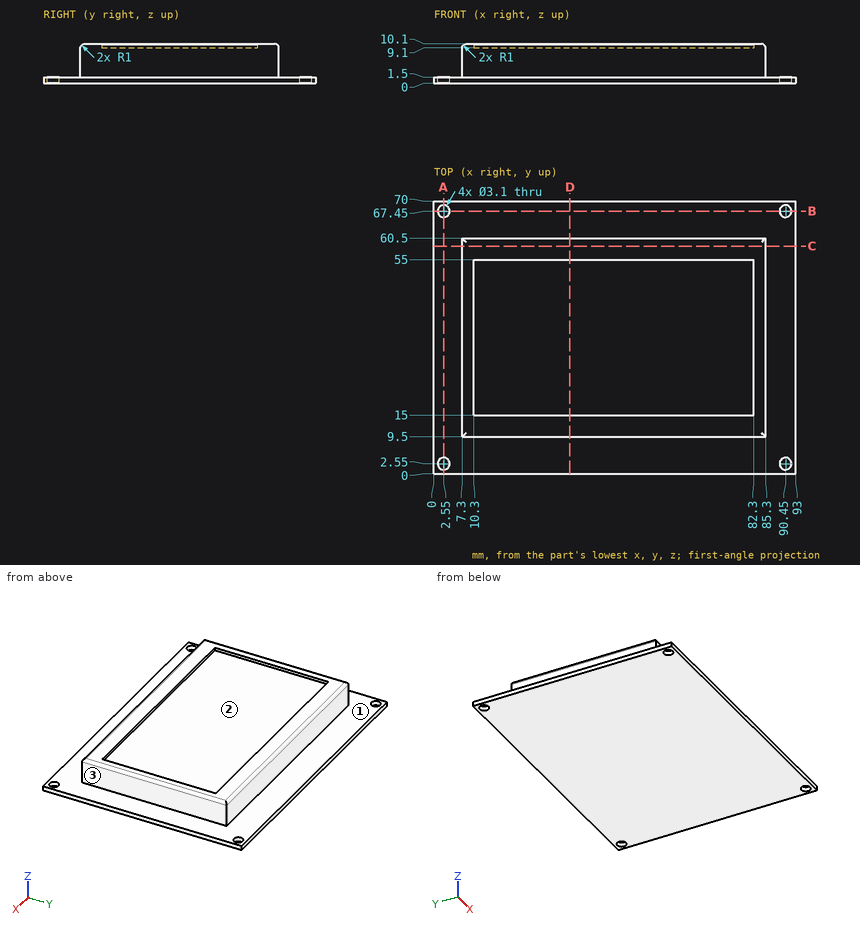
Job drawing, mm, ordinate dimensions from the low corner. One solid piece. Give positions to 0.01 mm unless a question says otherwise; leave off trailing zeros. Order: outer loops, then holes, each group sorted by start corner. A loop starts at its lowest first (then second) coordinate and runs counter-clockwise, first axis right, second up. Notation, with made-up numbers: (-1.75, -12.75) - (31.25, -12.75) arc R29 cw to (31.25, 25.25) - close; hole circle Ø8 at (23.25, -8.5). An arc over 180 degrees is marked (long way). Answer in a Markdown table with one row per item.
1. Saw through at B-B, the plane y = 67.45. Give the cut face in (x, z).
Data:
| item | result |
|---|---|
| outline | (0, 0) - (1, 0) - (1, 1.5) - (0, 1.5) - close; (4.1, 0) - (88.9, 0) - (88.9, 1.5) - (4.1, 1.5) - close; (92, 0) - (93, 0) - (93, 1.5) - (92, 1.5) - close |
2. Saw through at D-D, the plane x = 35. Give the cut face in (y, z).
Data:
| item | result |
|---|---|
| outline | (0, 0) - (70, 0) - (70, 1.5) - (60.5, 1.5) - (60.5, 9.1) arc R1 ccw to (59.5, 10.1) - (55, 10.1) - (55, 9.1) - (15, 9.1) - (15, 10.1) - (10.5, 10.1) arc R1 ccw to (9.5, 9.1) - (9.5, 1.5) - (0, 1.5) - close |
3. Flat gauge pins, fed straight in: pin 1 (4 mm diameter, centred on x = 90.45, y = 2.55, fed in from +Z); pin 2 (1 mm diameter, centred on x = 49, y = 46.5, fed in from +Z); pin 3 (6 mm diameter, centred on x = 59, z = 6.5, fed in from +Y); pin 4 (3 mm diameter, centred on x = 2.55, y = 67.45, fed in from +Z). Where does each tip first touch, or does it go through?
Data:
| item | result |
|---|---|
| pin 1 | stops at z = 1.5 |
| pin 2 | stops at z = 9.1 |
| pin 3 | stops at y = 60.5 |
| pin 4 | passes through |
4. Pull direction X, two halves, no side cores. Call the marked faces 1, 2 and 3: pulls with the +X half, pulls with the -X half, needs draft (parallel to the pull), parting line crosses it, or undercut.
Data:
| item | result |
|---|---|
| face 1 | needs draft |
| face 2 | undercut |
| face 3 | pulls with the +X half |
5. Saw through at A-A, the plane x = 2.55. Give the cut face in (y, z).
Data:
| item | result |
|---|---|
| outline | (0, 0) - (1, 0) - (1, 1.5) - (0, 1.5) - close; (4.1, 0) - (65.9, 0) - (65.9, 1.5) - (4.1, 1.5) - close; (69, 0) - (70, 0) - (70, 1.5) - (69, 1.5) - close |
6. Probe probe 1 along Y at (x, z) = (90.45, 0.6); probe 2 along Y at (x, z) = (44.5, 9.25); probe 3 along Z at (x, y) = (17, 34). List the from-to ranges inside material, lowest first. Write a range as [from, to].
Data:
| item | result |
|---|---|
| probe 1 | y = [0, 1], [4.1, 65.9], [69, 70] |
| probe 2 | y = [9.51, 15], [55, 60.49] |
| probe 3 | z = [0, 9.1] |
7. Saw through at C-C, the plane y = 58.5. Give the cut face in (x, z).
Data:
| item | result |
|---|---|
| outline | (0, 0) - (93, 0) - (93, 1.5) - (85.3, 1.5) - (85.3, 9.1) arc R1 ccw to (84.3, 10.1) - (8.3, 10.1) arc R1 ccw to (7.3, 9.1) - (7.3, 1.5) - (0, 1.5) - close |
